from build123d import *

# Parameters (mm, degrees)
BOSS_EXTRUDE2_DEPTH = 150
SKETCH4_W           = 21.1
SKETCH4_H           = 64.5
CUT_EXTRUDE1_DEPTH  = 1
SKETCH5_W           = 82
SKETCH5_H           = 41
CUT_EXTRUDE2_DEPTH  = 1
SKETCH6_W           = 140
SKETCH6_H           = 8
CUT_EXTRUDE3_DEPTH  = 3
SKETCH7_R           = 1.5
CUT_EXTRUDE4_DEPTH  = 3
SKETCH8_R           = 1.5
CUT_EXTRUDE5_DEPTH  = 3


with BuildPart() as part:
    # Sketch1 → Boss-Extrude2 (new body)
    with BuildSketch(Plane(origin=(0, 0, 0), x_dir=(0, 0, -1), z_dir=(1, 0, 0))):
        Polygon((-62.755935242, 0), (-62.755935242, 28), (-59.755935242, 28), (-59.755935242, 3), (17.244064758, 3), (17.244064758, 0), align=None)
    extrude(amount=-BOSS_EXTRUDE2_DEPTH)

    # Sketch4 → Cut-Extrude1 (cut)
    with BuildSketch(Plane(origin=(0, 3, 0), x_dir=(1, 0, 0), z_dir=(0, 1, 0))):
        with Locations((-139.45, -16.927076403)):
            Rectangle(SKETCH4_W, SKETCH4_H)
        with Locations((-10.55, -16.927076403)):
            Rectangle(SKETCH4_W, SKETCH4_H)
    extrude(amount=-CUT_EXTRUDE1_DEPTH, mode=Mode.SUBTRACT)

    # Sketch5 → Cut-Extrude2 (cut)
    with BuildSketch(Plane(origin=(0, 3, 0), x_dir=(1, 0, 0), z_dir=(0, 1, 0))):
        with Locations((-75, -4.705935242)):
            Rectangle(SKETCH5_W, SKETCH5_H)
    extrude(amount=-CUT_EXTRUDE2_DEPTH, mode=Mode.SUBTRACT)

    # Sketch6 → Cut-Extrude3 (cut)
    with BuildSketch(Plane.XY.offset(62.755935242)):
        with Locations((-75, 24)):
            Rectangle(SKETCH6_W, SKETCH6_H)
    extrude(amount=-CUT_EXTRUDE3_DEPTH, mode=Mode.SUBTRACT)

    # Sketch7 → Cut-Extrude4 (cut)
    with BuildSketch(Plane.XY.offset(62.755935242)):
        with Locations((-2.5, 25)):
            Circle(SKETCH7_R)
        with Locations((-147.5, 25)):
            Circle(SKETCH7_R)
    extrude(amount=-CUT_EXTRUDE4_DEPTH, mode=Mode.SUBTRACT)

    # Sketch8 → Cut-Extrude5 (cut)
    with BuildSketch(Plane(origin=(0, 3, 0), x_dir=(1, 0, 0), z_dir=(0, 1, 0))):
        with Locations(Location((-23.1, -47.755935242, 0), (0, 0, 270))):
            Circle(SKETCH8_R)
        with Locations(Location((-23.1, -20.005935242, 0), (0, 0, 270))):
            Circle(SKETCH8_R)
        with Locations(Location((-23.1, 7.744064758, 0), (0, 0, 270))):
            Circle(SKETCH8_R)
        with Locations(Location((-126.934112686, -47.755935242, 0), (0, 0, 270))):
            Circle(SKETCH8_R)
        with Locations(Location((-126.934112686, -20.005935242, 0), (0, 0, 270))):
            Circle(SKETCH8_R)
        with Locations(Location((-126.934112686, 7.744064758, 0), (0, 0, 270))):
            Circle(SKETCH8_R)
    extrude(amount=-CUT_EXTRUDE5_DEPTH, mode=Mode.SUBTRACT)


solid = part.part
Work out the finished part from the listing and answer in its coordinate system (mm). A direction names the side the tool comes from. Give positions to 0.01 mm unless a question says otherwise; leave off trailing zeros. Order: outer loops, then holes, each group sorted by start corner. A loop starts at its lowest first (then second) coordinate and runs counter-clockwise, first axis right, second up. Notation, with made-up numbers: (23.25, -9) - (72.25, -9) arc R23 cw to (72.25, 1) - close; hole circle Ø2 at (20, 19.25). An arc over 180 degrees is marked (long way). Answer as CSV lines item,"result". Start each with the question number.
Q1. The part is cut by section B-B (y = 25). Write down the section's boundary in (x, z), then the cut area to 3 significant figures.
Q2. The part is cut by section A-A (x = -2.5). Write down the section's boundary in (y, z).
Q3. Find the intervals of material crossed by L1, parallel to Y at x = -101.5, z = -5.5; L2, parallel to Y at x = -121, z = 21.5; L3, parallel to Z at x = -100.5, y = 5.25, in increasing order. Write a range as [from, to].
Q4. For faces 1 (the face through (-140, 2, 16)), 2 (the face through (-5, 24, 61)), 3 (the face through (-74, 13, 59.756)), determine the directions among +Z, -Z, +X, -X, +Y, -Y from which every point of the face is accessible in a straight line to the end or side of a thin tool.
Q5. Given pin 1 Ø4 at (y, z) = (5.5, 34.5) entering from -X (3 decimals); pin 2 Ø0.5 at (y, z) = (2.5, 27) entering from -X; pin 3 Ø8 at (x, z) = (-27.5, -2.5) entering from +Y; pin 4 Ø2.5 at (x, z) = (-47, 60.5) entering from +Y, each flat-ended and moving along its own axis, determine where each tip first touches the part or whether it passes through.
Q6. The part is cut by section C-C (z = 44). Write down the section's boundary in (x, y).
Q7. The part is cut by section D-D (x = -136). Write down the section's boundary in (y, z).
Q8. The mould has two halves that part along X. Classify faces 4 (the face through (-74, 3, 30)), 5 (the face through (0, 1.6, 34.4)), 6 (the face through (-76, 2, 4)): +X half, -X half, draft (parallel to the pull), parting line (faces both ways), or undercut.
Check result:
1,outline,"(-150, 59.76) - (-149, 59.76) - (-149, 62.76) - (-150, 62.76) - close; (-146, 59.76) - (-145, 59.76) - (-145, 62.76) - (-146, 62.76) - close; (-5, 59.76) - (-4, 59.76) - (-4, 62.76) - (-5, 62.76) - close; (-1, 59.76) - (0, 59.76) - (0, 62.76) - (-1, 62.76) - close"
1,area,"12.0 mm²"
2,outline,"(0, -17.24) - (3, -17.24) - (3, -15.32) - (2, -15.32) - (2, 49.18) - (3, 49.18) - (3, 59.76) - (23.5, 59.76) - (23.5, 62.76) - (0, 62.76) - close; (26.5, 59.76) - (28, 59.76) - (28, 62.76) - (26.5, 62.76) - close"
3,L1,"y = [0, 2]"
3,L2,"y = [0, 3]"
3,L3,"z = [59.76, 62.76]"
4,face 1,"-X, +Y"
4,face 2,"+Z, -Z, +Y"
4,face 3,"-Z, +X, -X, +Y"
5,pin 1,"passes through"
5,pin 2,"stops at x = -128.9"
5,pin 3,"stops at y = 3"
5,pin 4,"stops at y = 20"
6,outline,"(-150, 0) - (0, 0) - (0, 2) - (-21.1, 2) - (-21.1, 3) - (-128.9, 3) - (-128.9, 2) - (-150, 2) - close"
7,outline,"(0, -17.24) - (3, -17.24) - (3, -15.32) - (2, -15.32) - (2, 49.18) - (3, 49.18) - (3, 59.76) - (20, 59.76) - (20, 62.76) - (0, 62.76) - close"
8,face 4,"draft"
8,face 5,"+X half"
8,face 6,"undercut"
